Read the model definition and answer for the solid it produces. Units are mm, in the model's axes. A direction names the side the tool comes from. Give positions to 0.01 mm unless a question says otherwise; leave off trailing zeros. Write each loop counter-clockwise with the first axis right and the second up, starting at its lowest first coordinate (ties: lowest second). Pieces come first, ordered by that corner, then holes. Notation, with made-up numbers: (-4.5, 36.5) - (36.5, 36.5) arc R13 cw to (36.5, 57.5) - close; hole circle Ø11 at (-8.5, 89.5). An arc over 180 degrees is marked (long way). Answer as a JSON object with one key per item and string values. Group by question number.
Autodesk Inventor part; units mm, degrees
sketch "Sketch1" plane through (0, 0, 0) normal (0, 1, 0) x (-1, 0, 0)
  point P0 (0, 0)
sketch "Sketch2" plane through (0, 0, 0) normal (0, 1, 0) x (-1, 0, 0)
  circle A0 centre (0, 0) radius 1.25
  line L0 (60.55, 0) -> (-11.55, 0)
  line L1 (0, -71.35) -> (0, 13.35)
  circle A1 centre (49, 0) radius 1.25
  circle A2 centre (0, -58) radius 1.25
  circle A3 centre (49, -58) radius 1.25
  dimension "d0" = 2.5
  dimension "d3" = 49
  dimension "d6" = 58
extrude "Extrusion1" add sketch "Sketch2" along normal blind 10
sketch "Sketch3" plane through (0, 0, 0) normal (0, 1, 0) x (-1, 0, 0)
  line L0 (52.5, 3.5) -> (-3.5, 3.5)
  line L1 (-3.5, 3.5) -> (-3.5, -85)
  line L2 (-3.5, -85) -> (52.5, -85)
  line L3 (52.5, -85) -> (52.5, 3.5)
  circle A0 centre (49, 0) radius 1.25
  circle A1 centre (49, -58) radius 1.25
  circle A2 centre (0, 0) radius 1.25
  circle A3 centre (0, -58) radius 1.25
  line L4 (54.5, 5.5) -> (-5.5, 5.5)
  line L5 (-5.5, 5.5) -> (-5.5, -87)
  line L6 (-5.5, -87) -> (54.5, -87)
  line L7 (54.5, -87) -> (54.5, 5.5)
  dimension "d11" = 3.5
  dimension "d12" = 27
  dimension "d13" = 3.5
  dimension "d14" = 3.5
  dimension "d15" = 2
extrude "Extrusion2" add sketch "Sketch3" along normal blind 2 contours L3 L2 L1 L0 | L7 L6 L5 L4
sketch "Sketch4" plane through (0, 2, 0) normal (0, 1, 0) x (1, 0, 0)
  line L0 (-54.5, 87) -> (-54.5, -5.5)
  line L1 (-54.5, -5.5) -> (5.5, -5.5)
  line L2 (5.5, 87) -> (-54.5, 87)
  line L3 (5.5, -5.5) -> (5.5, 87)
  point P0 (0, 0)
sketch "Sketch5" plane through (0, 0, 0) normal (0, 0, 1) x (1, 0, 0)
  line L0 (-54.5, 0) -> (5.5, 0)
  line L1 (5.5, 0) -> (5.5, 2)
  line L2 (-54.5, 2) -> (5.5, 2)
  line L3 (-54.5, 0) -> (-54.5, 2)
  line L4 (5.5, 0) -> (7.5, 0)
  line L5 (7.5, 0) -> (7.5, 30)
  line L6 (7.5, 30) -> (5.5, 30)
  line L7 (5.5, 30) -> (5.5, 0)
  point P0 (0, 0)
  dimension "d18" = 2
  dimension "d19" = 30
sketch3d "3D Sketch1"
sketch3d "3D Sketch2"
  line L0 (5.5, 2, -87) -> (5.5, 2, 5.5)
  line L1 (5.5, 2, 5.5) -> (-54.5, 2, 5.5)
  line L2 (-54.5, 2, 5.5) -> (-54.5, 2, -87)
sweep "Sweep2" add profiles "Sketch5" path "3D Sketch2" contours L1 L7 L6 L5 L4
sketch "Sketch6" plane through (7.5, 0, -87) normal (0, 0, -1) x (-1, 0, 0)
  line L0 (2, 30) -> (62, 30)
  line L1 (2, 30) -> (2, 2)
  line L2 (2, 25) -> (62, 25)
  line L3 (62, 30) -> (62, 2)
  line L4 (2, 25) -> (2, 2)
  line L5 (2, 2) -> (62, 2)
  line L6 (2, 2) -> (62, 2)
  line L7 (62, 25) -> (62, 2)
  line L8 (0, 0) -> (0, 30)
  line L9 (0, 30) -> (2, 30)
  line L10 (64, 0) -> (0, 0)
  line L11 (64, 0) -> (64, 30)
  line L12 (64, 30) -> (62, 30)
  point P0 (7.5, 0)
  dimension "d25" = 5
extrude "Extrusion3" add sketch "Sketch6" along normal blind 2 contours L0 L3 L2 L1 | L1 L5 L3 L12 L11 L10 L8 L9
sketch "Sketch8" plane through (-56.5, 30, 7.5) normal (0, 0, 1) x (1, 0, 0)
  line L0 (64, -30) -> (0, -30)
  line L1 (20, -30) -> (44, -30)
  line L2 (44, -30) -> (44, -25)
  line L3 (44, -25) -> (20, -25)
  line L4 (20, -25) -> (20, -30)
  line L5 (0, -30) -> (0, 0)
  line L6 (64, -30) -> (64, 0)
  point P0 (56.5, -30)
  dimension "d39" = 20
  dimension "d40" = 20
  dimension "d41" = 5
extrude "Extrusion5" cut sketch "Sketch8" against normal blind 2
sketch "Sketch9" plane through (0, 2, 0) normal (0, 1, 0) x (1, 0, 0)
  circle A0 centre (0, 0) radius 1.25
  circle A1 centre (0, 0) radius 1.25
  circle A2 centre (-49, 0) radius 1.25
  circle A3 centre (-49, 0) radius 1.25
  circle A4 centre (-49, 58) radius 1.25
  circle A5 centre (-49, 58) radius 1.25
  circle A6 centre (0, 58) radius 1.25
  circle A7 centre (0, 58) radius 1.25
  circle A8 centre (0, 58) radius 1.25
  circle A9 centre (0, 0) radius 2.5
  circle A10 centre (-49, 0) radius 1.25
  circle A11 centre (-49, 0) radius 2.5
  circle A12 centre (0, 58) radius 2.5
  circle A13 centre (-49, 58) radius 2.5
  dimension "d44" = 5
  dimension "d45" = 5
  dimension "d46" = 5
  dimension "d47" = 5
extrude "Extrusion6" add sketch "Sketch9" along normal blind 4
sketch "Sketch12" plane through (7.5, 0, -89) normal (0, 0, -1) x (-1, 0, 0)
  line L0 (10, 6) -> (5, 6)
  line L1 (5, 2) -> (10, 2)
  line L2 (10, 6) -> (5, 6)
  line L3 (2, 30) -> (10, 30)
  line L4 (10, 30) -> (10, 28)
  line L5 (10, 28) -> (2, 28)
  line L6 (2, 28) -> (2, 30)
  line L7 (2, 25) -> (62, 25)
  line L8 (2, 28) -> (10, 28)
  line L9 (10, 28) -> (10, 25)
  line L10 (10, 25) -> (2, 25)
  line L11 (2, 25) -> (2, 28)
  point P0 (7.5, 0)
  dimension "d72" = 8
  dimension "d73" = 2
sketch "Sketch13" plane through (7.5, 0, 7.5) normal (1, 0, 0) x (0, 0, -1)
  line L0 (2, 5) -> (2, 2)
  line L1 (2, 30) -> (2, 2)
  line L2 (2, 30) -> (2, 2)
  line L3 (2, 2) -> (2, 5)
  line L4 (63, 2) -> (68, 2)
  line L5 (5, 2) -> (10, 2)
  line L6 (5, 2) -> (10, 2)
  line L7 (63, 2) -> (68, 2)
  line L8 (2, 2) -> (96.5, 2)
  line L9 (96.5, 2) -> (2, 2)
  line L10 (94.5, 25) -> (94.5, 30)
  line L11 (96.5, 25) -> (96.5, 2)
  line L12 (4, 26.5) -> (92.5, 26.5)
  line L13 (92.5, 26.5) -> (92.5, 4)
  line L14 (92.5, 4) -> (4, 4)
  line L15 (4, 4) -> (4, 26.5)
  line L16 (96.5, 30) -> (0, 30)
  line L17 (96.5, 2) -> (96.5, 25)
  point P0 (7.5, 0)
  dimension "d67" = 2
  dimension "d68" = 2
  dimension "d69" = 3.5
  dimension "d70" = 2
extrude "Extrusion10" cut sketch "Sketch12" against normal up to surface (2 mm away) contours L5 L9 L7 L11
extrude "Extrusion11" cut sketch "Sketch13" against normal up to surface (2 mm away)
sketch "Sketch14" plane through (7.5, 0, -89) normal (0, 0, -1) x (-1, 0, 0)
  line L0 (64, 30) -> (66, 30)
  line L1 (66, 30) -> (66, 28)
  line L2 (66, 28) -> (64, 28)
  line L3 (64, 28) -> (64, 30)
  line L4 (66, 4) -> (64, 4)
  line L5 (64, 4) -> (64, 2)
  line L6 (64, 2) -> (66, 2)
  line L7 (66, 2) -> (66, 4)
  line L8 (64, 30) -> (0, 30)
  line L9 (64, 0) -> (64, 30)
  point P0 (7.5, 0)
  dimension "d78" = 2
  dimension "d79" = 2
  dimension "d80" = 2
  dimension "d81" = 2
  dimension "d82" = 0
  dimension "d83" = 0
  dimension "d84" = 0
  dimension "d85" = 24
extrude "Extrusion12" add sketch "Sketch14" against normal blind 94.5
ref_plane "Work Plane1" through (-24.5, 0, 7.5) normal (-1, 0, 0) x (0, 0, 1)
mirror "Mirror1" about plane through (-24.5, 0, 7.5) normal (-1, 0, 0) of "Extrusion12"
sketch "Sketch15" plane through (-56.5, 0, 7.5) normal (-1, 0, 0) x (0, 0, 1)
  line L0 (-4, 4) -> (-92.5, 4)
  line L1 (-92.5, 26.5) -> (-4, 26.5)
  line L2 (-4, 26.5) -> (-4, 4)
  line L3 (-92.5, 4) -> (-92.5, 26.5)
  point P0 (-7.5, 0)
extrude "Extrusion13" cut sketch "Sketch15" against normal blind 2
properties part number "PI_Skal_med_rals"
1) Find section B-B, the plane x = -18.5. Write down the section's boundary in (y, z).
2) Which of the six approach directions +Z, -Z, +X, -X, +Y, -Y give full straight-line access (tool end or side, diameter ignored) to faces 1 (the flat face through (9, 3, 5.5)), 2 (the flat face through (-49, 10, 0)), 3 (the flat face through (1, 6, -1)), 4 (the flat face through (-24, 5, 7)), 5 (the flat face through (7, 15, 3.5))?
3) Find the intervals of material crossed by line 1 (X direction, y = 3.5, z = -25.5); line 2 (X direction, y = 27.25, z = -4); line 3 (Z direction, x = -49.5, y = 3), in increasing order. Write a range as [from, to].
4) Find section D-D, the plane y = 20. Write down the section's boundary in (x, z), and give its area (3 significant figures).
5) Flat-ended cylindrical pins translate along their axes: pin 1 Ø1.6 at (y, z) = (26, -88.5) entering from +X; pin 2 Ø4 at (y, z) = (7.5, -55) entering from +X; pin 3 Ø1.6 at (x, y) = (-28.5, 0.5) entering from +Z. Find the tip coordinate at first contact, or state that the pin passes through.
6) For a pull along Y with two mould halves and no side action, classify faces 6 (the flat face through (-50, 6, 1)), 7 (the cylindrical face through (1.34, 3.97, -55.89)), 8 (the flat face through (-57, 4, -42)) as released by +Y, released by -Y, zero draft, split by the parting line, or undercut.
7) Find section A-A, the plane x = -41. Write down the section's boundary in (y, z).
8) Find section C-C, the plane z = -42. Write down the section's boundary in (x, y).
Values follow:
{
 "1": {"outline": "(0, -89) - (2, -89) - (2, 5.5) - (0, 5.5) - close; (5, 5.5) - (30, 5.5) - (30, 7.5) - (5, 7.5) - close; (25, -89) - (30, -89) - (30, -87) - (25, -87) - close"},
 "2": {"face 1": "+Z, +X, +Y, -Y", "face 2": "-Z, +X, -X, +Y", "face 3": "+Y", "face 4": "+Z, -Z, -Y", "face 5": "+X, -X"},
 "3": {"line 1": "x = [-58.5, -54.5], [5.5, 9.5]", "line 2": "x = [-56.5, -54.5], [5.5, 7.5]", "line 3": "z = [-60.45, -55.55], [-2.45, 2.45], [5.5, 7.5]"},
 "4": {"outline": "(-56.5, -89) - (-54.5, -89) - (-54.5, -85) - (-56.5, -85) - close; (-56.5, 3.5) - (-54.5, 3.5) - (-54.5, 5.5) - (5.5, 5.5) - (5.5, 3.5) - (7.5, 3.5) - (7.5, 7.5) - (-56.5, 7.5) - close; (5.5, -89) - (7.5, -89) - (7.5, -85) - (5.5, -85) - close", "area": "152 mm2"},
 "5": {"pin 1": "stops at x = 7.5", "pin 2": "stops at x = 1.85", "pin 3": "stops at z = 5.5"},
 "6": {"face 6": "released by +Y", "face 7": "zero draft", "face 8": "undercut"},
 "7": {"outline": "(0, -89) - (2, -89) - (2, 5.5) - (30, 5.5) - (30, 7.5) - (0, 7.5) - close; (25, -89) - (30, -89) - (30, -87) - (25, -87) - close"},
 "8": {"outline": "(-58.5, 2) - (-56.5, 2) - (-56.5, 0) - (7.5, 0) - (7.5, 2) - (9.5, 2) - (9.5, 4) - (5.5, 4) - (5.5, 2) - (-54.5, 2) - (-54.5, 4) - (-58.5, 4) - close; (-58.5, 28) - (-56.5, 28) - (-56.5, 26.5) - (-54.5, 26.5) - (-54.5, 30) - (-58.5, 30) - close; (5.5, 26.5) - (7.5, 26.5) - (7.5, 28) - (9.5, 28) - (9.5, 30) - (5.5, 30) - close"}
}
